```python
from build123d import *

# Parameters (mm, degrees)
SKETCH1_R           = 100
BOSS_EXTRUDE1_DEPTH = 350
SKETCH2_R           = 125
SKETCH2_R_2         = 100
BOSS_EXTRUDE2_DEPTH = 100


with BuildPart() as part:
    # Sketch1 → Boss-Extrude1 (new body)
    with BuildSketch(Plane.XY):
        with BuildLine():
            Line((-125, 175), (125, 175))
            ThreePointArc((125, 175), (160.355339059, 160.355339059), (175, 125))
            Line((175, 125), (175, -125))
            ThreePointArc((175, -125), (160.355339059, -160.355339059), (125, -175))
            Line((125, -175), (-125, -175))
            ThreePointArc((-125, -175), (-160.355339059, -160.355339059), (-175, -125))
            Line((-175, -125), (-175, 125))
            ThreePointArc((-175, 125), (-160.355339059, 160.355339059), (-125, 175))
        make_face()
        Circle(SKETCH1_R, mode=Mode.SUBTRACT)
    extrude(amount=BOSS_EXTRUDE1_DEPTH)

    # Sketch2 → Boss-Extrude2 (add)
    with BuildSketch(Plane(origin=(0, 175, 0), x_dir=(1, 0, 0), z_dir=(0, 1, 0))):
        with Locations(Location((0, -175, 0), (0, 0, 180))):
            Circle(SKETCH2_R)
        with Locations(Location((0, -175, 0), (0, 0, 270))):
            Circle(SKETCH2_R_2, mode=Mode.SUBTRACT)
    extrude(amount=BOSS_EXTRUDE2_DEPTH)


solid = part.part
```
Verification items for the finished model (mm, model axes). A direction names the side the tool comes from. Give positions to 0.01 mm unless a question says otherwise; leave off trailing zeros. Loops run counter-clockwise (first coordinate to the right, second up) from the corner with the lowest first, then second, coordinate; pieces in that order, holes last. Notation, with made-up numbers: M 72,89.25 L 89,89.25 A17 cw 89,122.25 Z; hole C 72.25,4.5 d8. An arc over 180 degrees is marked long. Return JSON: item names as keys, results as strings.
1) Tool access check on faces 1 (the cylindrical face through (27.098, 224.3, 52.972)), 2 (the flat face through (175, 2, 173)). Record the directions out of +Z, -Z, +X, -X, +Y, -Y that give a thin tool (end or side, any length) a straight path to the whole face; none if there is none.
Findings:
{"face 1": "+Y", "face 2": "+Z, -Z, +X, +Y, -Y"}
2) Section check C-C, the plane z = 148.5. Enter the section's corners in (x, y), and give its area (3 significant figures).
Findings:
{"outline": "M -175,-125 A50 ccw -125,-175 L 125,-175 A50 ccw 175,-125 L 175,125 A50 ccw 125,175 L 122.16,175 L 122.16,275 L 96.42,275 L 96.42,175 L -96.42,175 L -96.42,275 L -122.16,275 L -122.16,175 L -125,175 A50 ccw -175,125 Z; hole C 0,0 d200", "area": "94,100 mm2"}
3) Gauge pin test, flat ends, axial feed: P1, Ø5, axis at x = -24.5, z = 145, coming from the +Y side; P2, Ø12, axis at x = -21, y = 87.5, coming from the +Z side. Record the tip position at first contact, or that the pin passes through.
Findings:
{"P1": "stops at y = 175", "P2": "passes through"}
4) Section check A-A, the plane x = 0. Enter the section's corners in (y, z).
Findings:
{"outline": "M -175,0 L -100,0 L -100,350 L -175,350 Z; M 100,0 L 175,0 L 175,50 L 275,50 L 275,75 L 175,75 L 175,275 L 275,275 L 275,300 L 175,300 L 175,350 L 100,350 Z"}
5) Material ranges on L1, parallel to X at y = -3, z = 219; L2, parallel to Y at x = 87, z = 263; L3, parallel to Y at x = 0, z = 276, recorded low to high. Write a range as [from, to].
Findings:
{"L1": "x = [-175, -99.95], [99.95, 175]", "L2": "y = [-175, -49.31], [49.31, 275]", "L3": "y = [-175, -100], [100, 275]"}
6) Section check B-B, the plane y = 0. Enter the section's corners in (x, z).
Findings:
{"outline": "M -175,0 L -100,0 L -100,350 L -175,350 Z; M 100,0 L 175,0 L 175,350 L 100,350 Z"}
7) Mould release check, pull along Z, two halves, no side actions. Record for faces 3 (the cylindrical face through (30.04, 224.3, 270.38)), 4 (the flat face through (-1, 175, 174)), 5 (the cylindrical face through (160.742, -159.964, 172.55)), 6 (the flat face through (80, -75, 350)): released by +Z, released by -Z, zero draft, split by the parting line, or undercut.
Findings:
{"face 3": "undercut", "face 4": "undercut", "face 5": "zero draft", "face 6": "released by +Z"}
8) Section check D-D, the plane x = -39. Enter the section's corners in (y, z), and give its area (3 significant figures).
Findings:
{"outline": "M -175,0 L -92.08,0 L -92.08,350 L -175,350 Z; M 92.08,0 L 175,0 L 175,56.24 L 275,56.24 L 275,82.92 L 175,82.92 L 175,267.08 L 275,267.08 L 275,293.76 L 175,293.76 L 175,350 L 92.08,350 Z", "area": "63,400 mm2"}
